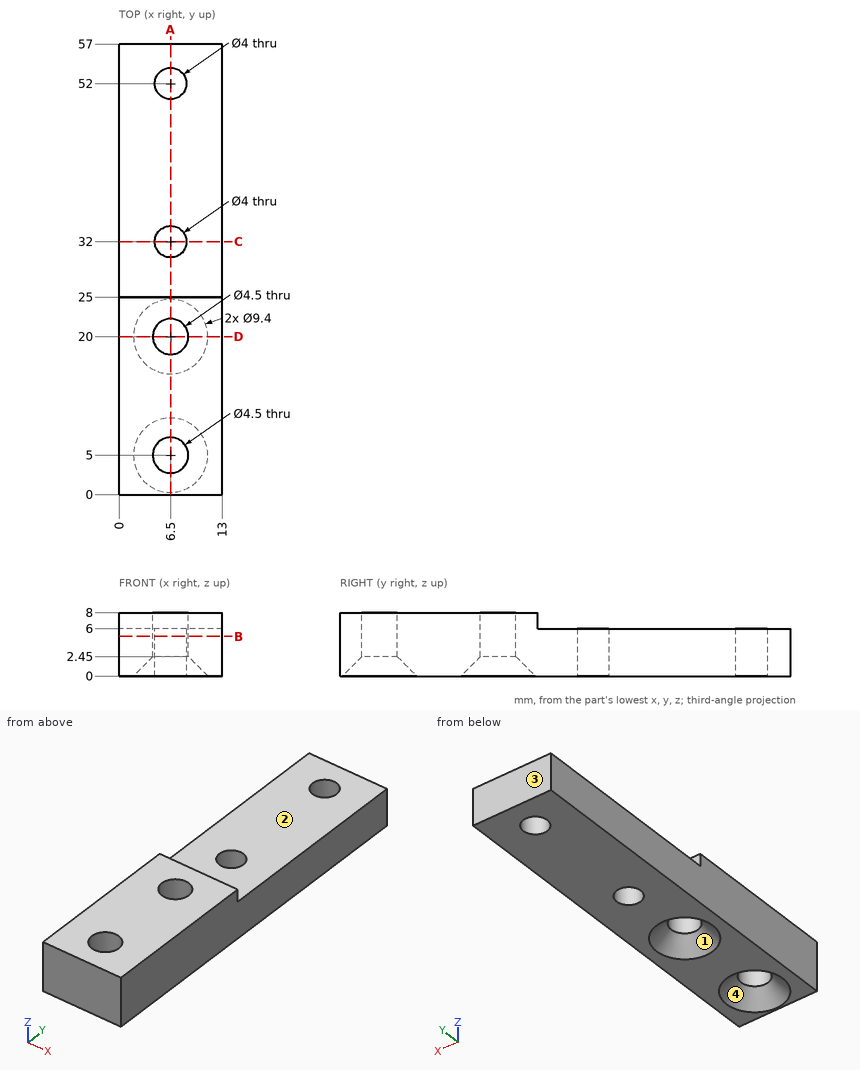
Verification items for this drawing (mm, ordinates from the low corner). Give positions to 0.01 mm unless a question says otherwise; leave off trailing zeros. Write each loop counter-clockwise with the first axis right and the second up, starting at its lowest first coordinate (ties: lowest second). Pieces come first, ordered by that corner, then holes.
1) Cross-section at A-A (x = 6.5). Record the boundary of the cut face in (y, z), plus the area to 3 significant figures.
Values follow:
outline: (0, 0) - (0.3, 0) - (2.75, 2.45) - (2.75, 8) - (0, 8) - close; (7.25, 2.45) - (9.7, 0) - (15.3, 0) - (17.75, 2.45) - (17.75, 8) - (7.25, 8) - close; (22.25, 2.45) - (24.7, 0) - (30, 0) - (30, 6) - (25, 6) - (25, 8) - (22.25, 8) - close; (34, 0) - (50, 0) - (50, 6) - (34, 6) - close; (54, 0) - (57, 0) - (57, 6) - (54, 6) - close
area: 260 mm2
2) Thickness scan on line 1 (Y direction, x = 6.5, z = 6.55); line 2 (Y direction, x = 6.5, z = 5.05); line 3 (X direction, y = 20, z = 5.6). Record the ranges inside material, lowest first.
Values follow:
line 1: y = 0 to 2.75, 7.25 to 17.75, 22.25 to 25
line 2: y = 0 to 2.75, 7.25 to 17.75, 22.25 to 30, 34 to 50, 54 to 57
line 3: x = 0 to 4.25, 8.75 to 13
3) Release check for a two-part mould opening along Y. For the marked faces 1, 2, 3 and 4 record: released by +Y, released by -Y, zero draft, split by the parting line, or undercut.
Values follow:
face 1: undercut
face 2: zero draft
face 3: released by +Y
face 4: undercut
4) Cross-section at C-C (y = 32). Record the boundary of the cut face in (x, z), plus the area to 3 significant figures.
Values follow:
outline: (0, 0) - (4.5, 0) - (4.5, 6) - (0, 6) - close; (8.5, 0) - (13, 0) - (13, 6) - (8.5, 6) - close
area: 54.0 mm2
5) Cross-section at D-D (y = 20). Record the boundary of the cut face in (x, z), plus the area to 3 significant figures.
Values follow:
outline: (0, 0) - (1.8, 0) - (4.25, 2.45) - (4.25, 8) - (0, 8) - close; (8.75, 2.45) - (11.2, 0) - (13, 0) - (13, 8) - (8.75, 8) - close
area: 62.0 mm2
6) Cross-section at B-B (z = 5). Record the boundary of the cut face in (x, y), plus the area to 3 significant figures.
Values follow:
outline: (0, 0) - (13, 0) - (13, 57) - (0, 57) - close; hole circle Ø4.5 at (6.5, 5); hole circle Ø4.5 at (6.5, 20); hole circle Ø4 at (6.5, 32); hole circle Ø4 at (6.5, 52)
area: 684 mm2
